from build123d import *

# Parameters (mm, degrees)
F0_R     = 3
F0_R_2   = 5
F1_DEPTH = 15


with BuildPart() as f1:
    # F0 (on Front) → F1 (new body)
    with BuildSketch(Plane.XZ):
        with BuildLine():
            Line((-25.619237, 119.997091), (-26.454732, 0))
            Line((-26.454732, 0), (133.545268, 0))
            Line((133.545268, 0), (133.545268, 200))
            ThreePointArc((133.545268, 200), (113.545268, 220), (93.545268, 200))
            Line((93.545268, 200), (93.545268, 143.251527))
            ThreePointArc((93.545268, 143.251527), (90.000959, 134.736758), (81.461719, 131.251818))
            Line((81.461719, 131.251818), (-13.535978, 131.913251))
            ThreePointArc((-13.535978, 131.913251), (-22.045525, 128.457696), (-25.619237, 119.997091))
        make_face()
        with BuildLine():
            Line((98.498465, 88.689308), (98.498465, 98.683833))
            ThreePointArc((98.498465, 98.683833), (112.620812, 85.723137), (126.441521, 99.005017))
            Line((126.441521, 99.005017), (126.441521, 23.286659))
            ThreePointArc((126.441521, 23.286659), (122.926803, 14.801378), (114.441521, 11.286659))
            Line((114.441521, 11.286659), (0.203851, 11.286659))
            ThreePointArc((0.203851, 11.286659), (-8.281431, 14.801378), (-11.796149, 23.286659))
            Line((-11.796149, 23.286659), (-11.796149, 64.689308))
            ThreePointArc((-11.796149, 64.689308), (-8.281431, 73.174589), (0.203851, 76.689308))
            Line((0.203851, 76.689308), (86.498465, 76.689308))
            ThreePointArc((86.498465, 76.689308), (94.983746, 80.204026), (98.498465, 88.689308))
        make_face(mode=Mode.SUBTRACT)
        with Locations((-13.619528, 119.913542)):
            Circle(F0_R, mode=Mode.SUBTRACT)
        with Locations((113.545268, 200)):
            Circle(F0_R_2, mode=Mode.SUBTRACT)
    extrude(amount=F1_DEPTH)


solid = f1.part
Build history of the part. All positions in model axes, mm. A direction names the side the tool comes from. Coordinates: 2 decimals unless noted, no trailing zeros. Order: outer loops, then holes, each group sorted by start corner. A loop starts at its lowest first (then second) coordinate and runs counter-clockwise, first axis right, second up. Notation, with made-up numbers: (32, 2) - (58, 2) arc R20 cw to (58, 31) - close; hole circle Ø9 at (-16, -40). An arc over 180 degrees is marked (long way). Put each result on its own line as item: value.
1. Saw through at C-C (y = -2.75). Write the cut outline in (x, z), and give its area (3 significant figures).
Answer sheet:
outline: (-26.45, 0) - (133.55, 0) - (133.55, 200) arc R20 ccw to (93.55, 200) - (93.55, 143.25) arc R12 cw to (81.46, 131.25) - (-13.54, 131.91) arc R12 ccw to (-25.62, 120) - close; hole circle Ø6 at (-13.62, 119.91); hole (-11.8, 23.29) arc R12 ccw to (0.2, 11.29) - (114.44, 11.29) arc R12 ccw to (126.44, 23.29) - (126.44, 99.01) arc R14 cw to (98.5, 98.68) - (98.5, 88.69) arc R12 cw to (86.5, 76.69) - (0.2, 76.69) arc R12 ccw to (-11.8, 64.69) - close; hole circle Ø10 at (113.55, 200)
area: 14,900 mm^2
2. Drop flat-ended pins along their axis: P1, Ø7.5, axis at x = 35.5, y = -4, coming from the -Z side; P2, Ø3, axis at x = 0.5, y = -10.5, coming from the +Z side; P3, Ø4.5, axis at y = -9.5, z = 159, coming from the -X side. Give the stop position or say it passes through.
Answer sheet:
P1: stops at z = 0
P2: stops at z = 131.83
P3: stops at x = 93.55
3. Saw through at D-D (z = 159). Write the cut outline in (x, y).
Answer sheet:
outline: (93.55, -15) - (133.55, -15) - (133.55, 0) - (93.55, 0) - close
4. Saw through at B-B (z = 83.5). Write the cut outline in (x, y).
Answer sheet:
outline: (-25.87, -15) - (97.32, -15) - (97.32, 0) - (-25.87, 0) - close; (126.44, -15) - (133.55, -15) - (133.55, 0) - (126.44, 0) - close
5. Pull direction Z, two halves, no side cores. Call faces 1 (the face through (123.02, -7.395, 14.895)), 2 (the face through (90.094, -7.395, 134.831)), 3 (the face through (52, -7, 0)): pulls with the +Z half, pulls with the -Z half, needs draft (parallel to the pull), parting line crosses it, or undercut.
Answer sheet:
face 1: undercut
face 2: pulls with the +Z half
face 3: pulls with the -Z half
6. Saw through at A-A (x = 63). Write the cut outline in (y, z), and give its area (3 significant figures).
Answer sheet:
outline: (-15, 0) - (0, 0) - (0, 11.29) - (-15, 11.29) - close; (-15, 76.69) - (0, 76.69) - (0, 131.38) - (-15, 131.38) - close
area: 990 mm^2
7. Tool access for faces 4 (the face through (43, -7, 76.689)), 5 (the face through (93.545, -7, 172)), 6 (the face through (133.545, -7, 99)): list every direction of +Z, -Z, +X, -X, +Y, -Y with a clear straight run to the whole face (end or side of a thin tool).
Answer sheet:
face 4: +Y, -Y
face 5: +Z, -X, +Y, -Y
face 6: +Z, -Z, +X, +Y, -Y
8. Probe line 1 along Z through (x, y) = (79.5, -9.75); line 2 along Z through (x, y) = (117.5, -1.5); line 3 along Z through (x, y) = (109.5, -12.5). List the from-to ranges inside material, lowest first. Write a range as [from, to].
Answer sheet:
line 1: z = [0, 11.29], [76.69, 131.27]
line 2: z = [0, 11.68], [86.66, 196.94], [203.06, 219.61]
line 3: z = [0, 11.29], [86.04, 197.06], [202.94, 219.59]
